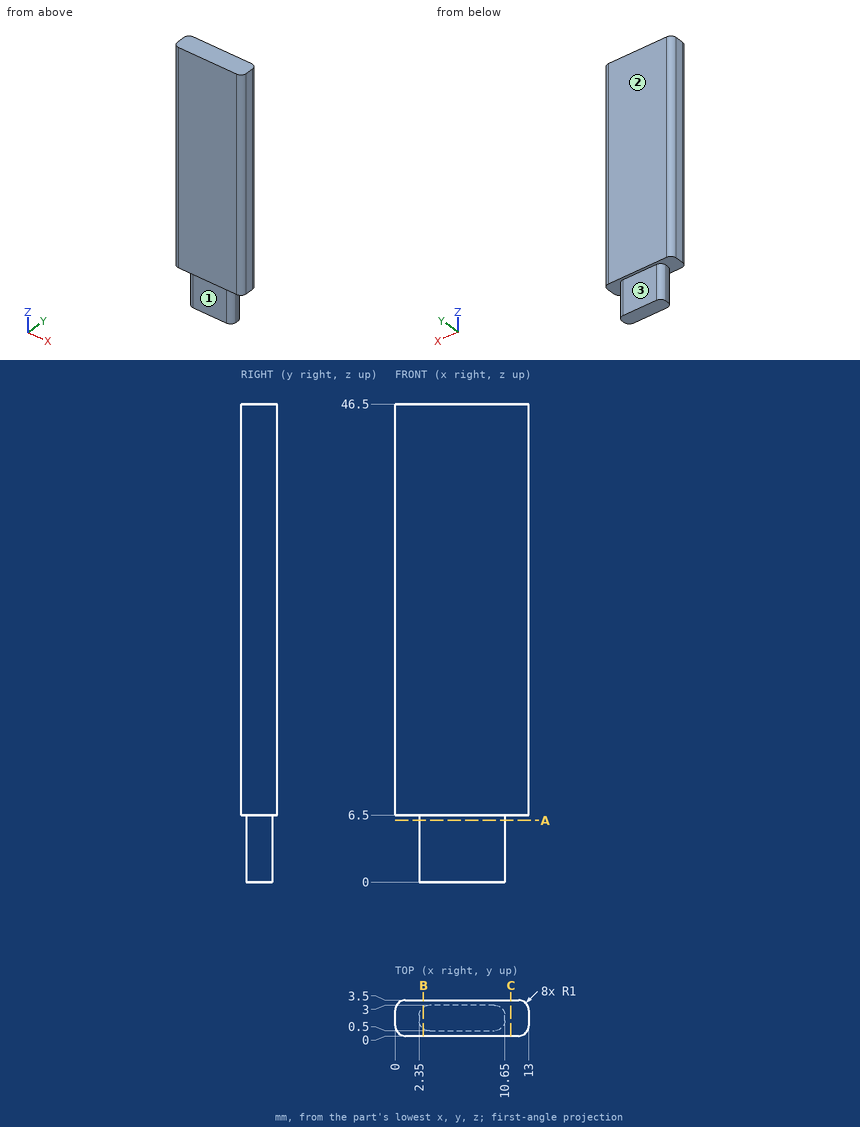
Can you work these out from the drawing? Everything is in mm from the part's minimum corner. A direction names the side the tool comes from. Round coordinates to 2 decimals unless told otherwise and drop trailing zeros. Loops run counter-clockwise (first coordinate to the right, second up) from the corner with the lowest first, then second, coordinate; pieces in that order, holes last. Notation, with made-up numbers: (-19.75, 24.25) - (1.25, 24.25) arc R6 ccw to (1.25, 33.25) - close; hole circle Ø10 at (50, -21.5). An arc over 180 degrees is marked (long way). One line per question, with ' | ' between items. Start each with the question number.
Q1. I want a section at C-C (x = 11.25). Write out the boundary of the cut face in (y, z).
Q2. I want a section at A-A (z = 6). Write out the boundary of the cut face in (x, y), then the cut area to 3 significant figures.
Q3. Will these pins go through, and if not, where does the flat tip stop? pin 1 (3 mm diameter, centred on x = 7, z = 3.5, fed in from -Y); pin 2 (1.9 mm diameter, centred on x = 5, z = 4, fed in from +Y); pin 3 (0.6 mm diameter, centred on y = 1.5, z = 3.5, fed in from -X).
Q4. For the marked faces 1, 2 and 3, which set-ups out of +Z, -Z, +X, -X, +Y, -Y let a thin tool reach every point of the face, with its end or its side?
Q5. I want a section at B-B (x = 2.75). Write out the boundary of the cut face in (y, z), then the cut area to 3 significant figures.
Q6. Please list where these lines run through material, in increasing order: line 1 (Z direction, x = 2.5, y = 0.9); line 2 (X direction, y = 1.65, z = 3.5); line 3 (X direction, y = 1.4, z = 4). Write a range as [from, to].
Response values:
1) outline: (0, 6.5) - (3.5, 6.5) - (3.5, 46.5) - (0, 46.5) - close
2) outline: (2.35, 1.5) arc R1 ccw to (3.35, 0.5) - (9.65, 0.5) arc R1 ccw to (10.65, 1.5) - (10.65, 2) arc R1 ccw to (9.65, 3) - (3.35, 3) arc R1 ccw to (2.35, 2) - close | area: 19.9 mm²
3) pin 1: stops at y = 0.5 | pin 2: stops at y = 3 | pin 3: stops at x = 2.35
4) face 1: -Z, +X, -X, -Y | face 2: +Z, -Z, +X, -X, +Y | face 3: -Z, +X, -X, +Y
5) outline: (0, 6.5) - (0.7, 6.5) - (0.7, 0) - (2.8, 0) - (2.8, 6.5) - (3.5, 6.5) - (3.5, 46.5) - (0, 46.5) - close | area: 154 mm²
6) line 1: z = [6.5, 46.5] | line 2: x = [2.35, 10.65] | line 3: x = [2.36, 10.64]
